from build123d import *

# Parameters (mm, degrees)
SKETCH1_R           = 7.239
BOSS_EXTRUDE1_DEPTH = 7.62
SKETCH2_R           = 23.495
SKETCH2_R_2         = 15.875
BOSS_EXTRUDE2_DEPTH = 80.01
FILLET1_R           = 2.54
SKETCH4_R           = 5.08
CUT_EXTRUDE1_DEPTH  = 80.01


with BuildPart() as part:
    # Sketch1 → Boss-Extrude1 (new body)
    with BuildSketch(Plane(origin=(0, 0, 0), x_dir=(1, 0, 0), z_dir=(0, 1, 0))):
        with BuildLine():
            Line((-49.022, 35.052), (49.022, 35.052))
            ThreePointArc((49.022, 35.052), (84.074, 0), (49.022, -35.052))
            Line((49.022, -35.052), (-49.022, -35.052))
            ThreePointArc((-49.022, -35.052), (-84.074, 0), (-49.022, 35.052))
        make_face()
        with Locations(Location((-49.022, 0, 0), (0, 0, 90))):
            Circle(SKETCH1_R, mode=Mode.SUBTRACT)
        with Locations(Location((49.022, 0, 0), (0, 0, 90))):
            Circle(SKETCH1_R, mode=Mode.SUBTRACT)
        with Locations(Location((0, 0, 0), (0, 0, 90))):
            Circle(SKETCH1_R, mode=Mode.SUBTRACT)
    extrude(amount=BOSS_EXTRUDE1_DEPTH)

    # Sketch2 → Boss-Extrude2 (add)
    with BuildSketch(Plane(origin=(0, 7.62, 0), x_dir=(1, 0, 0), z_dir=(0, 1, 0))):
        with Locations(Location((0, 0, 0), (0, 0, 270))):
            Circle(SKETCH2_R)
        with Locations(Location((0, 0, 0), (0, 0, 270))):
            Circle(SKETCH2_R_2, mode=Mode.SUBTRACT)
    extrude(amount=BOSS_EXTRUDE2_DEPTH)

    # Fillet1
    fillet1_edges = [part.edges().sort_by_distance(p)[0] for p in [
        (84.074, 7.62, 0),
        (0, 7.62, -35.052),
        (0, 87.63, -23.495),
        (-84.074, 7.62, 0),
        (0, 7.62, 35.052),
    ]]
    fillet(fillet1_edges, radius=FILLET1_R)

    # Sketch4 → Cut-Extrude1 (cut)
    with BuildSketch(Plane.XY):
        with Locations(Location((0, 60.96, 0), (0, 0, 180))):
            Circle(SKETCH4_R)
        with Locations(Location((0, 30.48, 0), (0, 0, 180))):
            Circle(SKETCH4_R)
    extrude(amount=CUT_EXTRUDE1_DEPTH, mode=Mode.SUBTRACT)


solid = part.part
Part model, mm, in its own coordinate system. A direction names the side the tool comes from. Coordinates: 2 decimals unless noted, no trailing zeros. Order: outer loops, then holes, each group sorted by start corner. A loop starts at its lowest first (then second) coordinate and runs counter-clockwise, first axis right, second up.
(1) Slice it at B-B, the plane z = 0. Write the cut outline in (x, y) (3 decimals), and give its area (3 significant figures).
Check sheet entries:
outline: (-84.074, 0) - (-56.261, 0) - (-56.261, 7.62) - (-81.534, 7.62) arc R2.54 ccw to (-84.074, 5.08) - close; (-41.783, 0) - (-7.239, 0) - (-7.239, 7.62) - (-15.875, 7.62) - (-15.875, 87.63) - (-20.955, 87.63) arc R2.54 ccw to (-23.495, 85.09) - (-23.495, 7.62) - (-41.783, 7.62) - close; (7.239, 0) - (41.783, 0) - (41.783, 7.62) - (23.495, 7.62) - (23.495, 85.09) arc R2.54 ccw to (20.955, 87.63) - (15.875, 87.63) - (15.875, 7.62) - (7.239, 7.62) - close; (56.261, 0) - (84.074, 0) - (84.074, 5.08) arc R2.54 ccw to (81.534, 7.62) - (56.261, 7.62) - close
area: 2,160 mm2
(2) Probe L1, parallel to Y at x = 0, z = 17.5; L2, parallel to X at y = 2, z = 0; L3, parallel to X at y = 18, z = 1. List the from-to ranges inside material, lowest first.
Check sheet entries:
L1: y = 0 to 25.4, 35.56 to 55.88, 66.04 to 87.63
L2: x = -84.07 to -56.26, -41.78 to -7.24, 7.24 to 41.78, 56.26 to 84.07
L3: x = -23.47 to -15.84, 15.84 to 23.47
(3) Slice it at C-C, the plane x = 38. Write the cut outline in (y, z).
Check sheet entries:
outline: (0, -35.05) - (5.08, -35.05) arc R2.54 ccw to (7.62, -32.51) - (7.62, 32.51) arc R2.54 ccw to (5.08, 35.05) - (0, 35.05) - close
(4) Slice it at D-D, the plane y = 73.5. Write the cut outline in (x, z) (3 decimals), and give its area (3 significant figures).
Check sheet entries:
outline: circle Ø46.99 at (0, 0); hole circle Ø31.75 at (0, 0)
area: 942 mm2
(5) Pull direction Y, two halves, no side cores. Call faces 4 (the face through (7.067, 3.757, 1.569)), 5 (the face through (1, 0, -8)), 6 (the face through (-4.845, 59.434, 19.208)), 7 (the face through (-7, 7.62, 3)): pulls with the +Y half, pulls with the -Y half, needs draft (parallel to the pull), parting line crosses it, or undercut.
Check sheet entries:
face 4: needs draft
face 5: pulls with the -Y half
face 6: undercut
face 7: pulls with the +Y half
(6) Tool access for faces 1 (the face through (-4.69, 32.43, 19.21)), 2 (the face through (-22.936, 45.813, -5.093)), 3 (the face through (-84.066, 2.504, 0.771)): list every direction of +Z, -Z, +X, -X, +Y, -Y with a clear straight run to the whole face (end or side of a thin tool).
Check sheet entries:
face 1: +Z
face 2: +Y
face 3: -X, +Y, -Y
(7) Pin check, flat tips, straight feed: pin 1 Ø9.5 at (x, z) = (4.5, -1) entering from +Y; pin 2 Ø1.5 at (y, z) = (52.5, -9) entering from +X; pin 3 Ø1 at (x, y) = (13.5, 34.5) entering from -Z. Stop position of each tip, or through.
Check sheet entries:
pin 1: stops at y = 7.62
pin 2: stops at x = 22
pin 3: stops at z = -19.57
(8) Slice it at A-A, the plane x = 0. Write the cut outline in (y, z) (3 decimals), and give its area (3 significant figures).
Check sheet entries:
outline: (0, -35.052) - (5.08, -35.052) arc R2.54 ccw to (7.62, -32.512) - (7.62, -23.495) - (85.09, -23.495) arc R2.54 ccw to (87.63, -20.955) - (87.63, -15.875) - (7.62, -15.875) - (7.62, -7.239) - (0, -7.239) - close; (0, 7.239) - (7.62, 7.239) - (7.62, 15.875) - (25.4, 15.875) - (25.4, 23.495) - (7.62, 23.495) - (7.62, 32.512) arc R2.54 ccw to (5.08, 35.052) - (0, 35.052) - close; (35.56, 15.875) - (55.88, 15.875) - (55.88, 23.495) - (35.56, 23.495) - close; (66.04, 15.875) - (87.63, 15.875) - (87.63, 20.955) arc R2.54 ccw to (85.09, 23.495) - (66.04, 23.495) - close
area: 1,480 mm2
